The figure shows three views and two pictorial views of one solid part (mm, origin at its lowest corner). Answer the questions. A direction names the side the tool comes from. Coordinates: 2 decimals unless noted, no trailing zeros. Write each loop counter-clockwise with the first axis right and the second up, starting at its lowest first coordinate (ties: lowest second). Pieces come first, ordered by that corner, then holes.
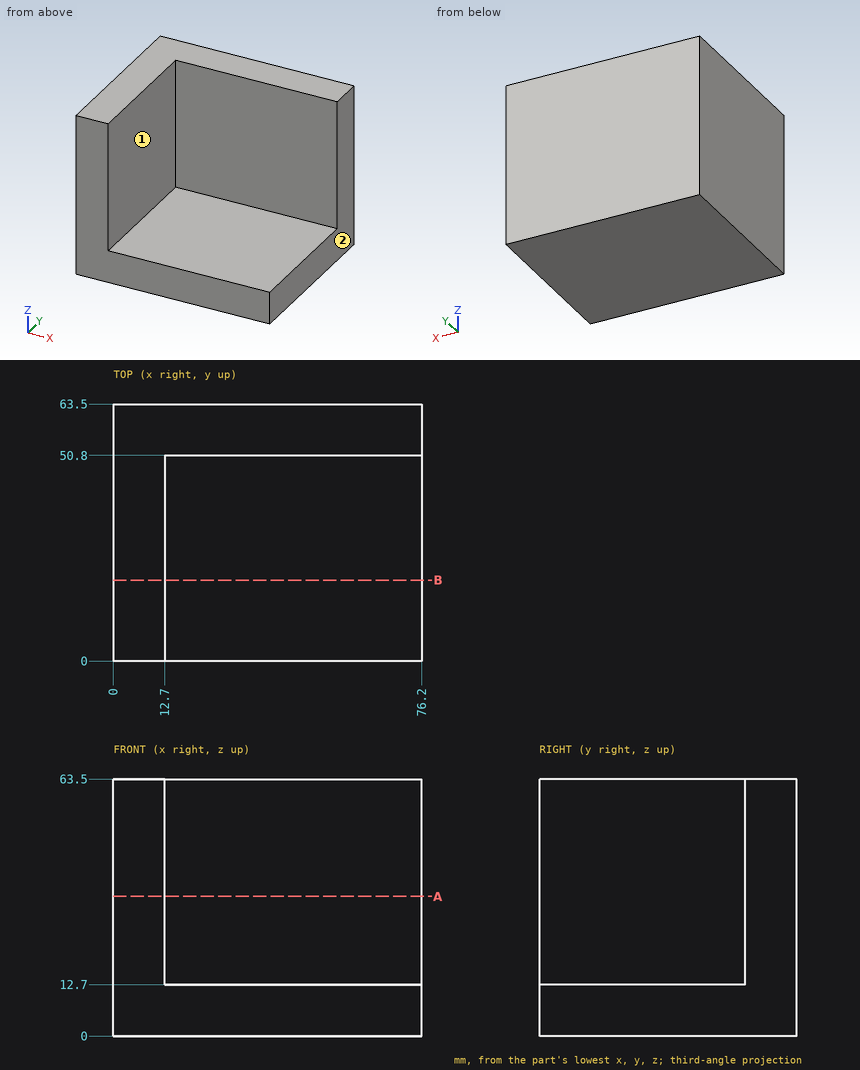
1. Flat-ended cylindrical pins translate along their axes: P1, Ø1, axis at y = 49.5, z = 46, coming from the +X side; P2, Ø6, axis at x = 52, y = 23, coming from the +Z side. Find the tip coordinate at first contact, or state that the pin passes through.
Results found:
P1: stops at x = 12.7
P2: stops at z = 12.7
2. Section A-A on z = 34.5 is taken. Give the vertices of the cut face in (x, y).
Results found:
outline: (0, 0) - (12.7, 0) - (12.7, 50.8) - (76.2, 50.8) - (76.2, 63.5) - (0, 63.5) - close
3. Find the intervals of material crossed by L1, parallel to Y at x = 37, z = 15.5; L2, parallel to X at y = 4, z = 59, in increasing order.
Results found:
L1: y = 50.8 to 63.5
L2: x = 0 to 12.7
4. A tool of negligible diameter and unlimited length cuts with its end or side. For the marked faces 1 and 2, from which of +Z, -Z, +X, -X, +Y, -Y can it reach the whole face along a straight path? Write none if from no direction.
Results found:
face 1: +Z, +X, -Y
face 2: +Z, -Z, +X, +Y, -Y
5. Section B-B on y = 20 is taken. Give the vertices of the cut face in (x, z), then the cut area to 3 significant figures.
Results found:
outline: (0, 0) - (76.2, 0) - (76.2, 12.7) - (12.7, 12.7) - (12.7, 63.5) - (0, 63.5) - close
area: 1,610 mm2
